```python
from build123d import *

# Parameters (mm, degrees)
SKETCH1_R            = 19
BOSS_EXTRUDE1_DEPTH  = 9.525
M5_CLEARANCE_HOLE1_D = 5.3


with BuildPart() as part:
    # Sketch1 → Boss-Extrude1 (new body)
    with BuildSketch(Plane.XY):
        with Locations(Location((0, 0, 0), (0, 0, 180))):
            Circle(SKETCH1_R)
    extrude(amount=BOSS_EXTRUDE1_DEPTH)

    # M5 Clearance Hole1 (through all)
    with Locations(Plane.XY.offset(9.525)):
        with Locations((-11.919791467, 6.881894812), (0, 13.763789624), (11.919791467, 6.881894812), (11.919791467, -6.881894812), (0, -13.763789624), (-11.919791467, -6.881894812)):
            Hole(M5_CLEARANCE_HOLE1_D / 2)


solid = part.part
```
Here's how the part is built. I have some questions about the finished solid (model axes, mm). Round coordinates to 2 decimals unless told otherwise and drop trailing zeros. Write each loop counter-clockwise with the first axis right and the second up, starting at its lowest first coordinate (ties: lowest second). Pieces come first, ordered by that corner, then holes.
Q1. Will these pins go through, and if not, where does the flat tip stop? P1, Ø5, axis at x = -11.92, y = 6.88, coming from the +Z side; P2, Ø1.5, axis at y = 4.5, z = 1, coming from the +X side; P3, Ø3, axis at y = 11.5, z = 3, coming from the -X side.
Q2. If we section it at B-B on z = 6: Write out the boundary of the cut face in (x, y).
Q3. If we mould it in two halves opening along Y, with no side actions, what happens to faces 1 (the cylindrical face through (4.119, 18.548, 4.696)), 2 (the flat face through (0, 0, 9.525)), 3 (the cylindrical face through (0.57, -16.35, 4.7))? For each: +Y half, -Y half, draft (parallel to the pull), parting line (faces both ways), or undercut.
Q4. If we section it at D-D on x = 8: Write out the boundary of the cut face in (y, z) (3 decimals), plus the area to 3 significant figures.
Q5. If we section it at C-C on x = -11: Write out the boundary of the cut face in (y, z) (3 decimals).
Q6. Please list where these lines run through material, in increasing order: probe 1 along Y at (x, z) = (0, 7); probe 2 along X at (y, z) = (9, 4.5); probe 3 along Y at (x, z) = (-10, 6.25).
Q7. If we section it at A-A on x = 0: Write out the boundary of the cut face in (y, z) (3 decimals), plus the area to 3 significant figures.
Answer below:
1. P1: passes through
1. P2: stops at x = 18.63
1. P3: stops at x = -16.16
2. outline: circle Ø38 at (0, 0); hole circle Ø5.3 at (-11.92, -6.88); hole circle Ø5.3 at (-11.92, 6.88); hole circle Ø5.3 at (0, -13.76); hole circle Ø5.3 at (0, 13.76); hole circle Ø5.3 at (11.92, -6.88); hole circle Ø5.3 at (11.92, 6.88)
3. face 1: parting line
3. face 2: draft
3. face 3: undercut
4. outline: (-17.234, 0) - (17.234, 0) - (17.234, 9.525) - (-17.234, 9.525) - close
4. area: 328 mm2
5. outline: (-15.492, 0) - (-9.367, 0) - (-9.367, 9.525) - (-15.492, 9.525) - close; (-4.397, 0) - (4.397, 0) - (4.397, 9.525) - (-4.397, 9.525) - close; (9.367, 0) - (15.492, 0) - (15.492, 9.525) - (9.367, 9.525) - close
6. probe 1: y = -19 to -16.41, -11.11 to 11.11, 16.41 to 19
6. probe 2: x = -16.73 to -13.51, -10.33 to 10.33, 13.51 to 16.73
6. probe 3: y = -16.16 to -8.71, -5.06 to 5.06, 8.71 to 16.16
7. outline: (-19, 0) - (-16.414, 0) - (-16.414, 9.525) - (-19, 9.525) - close; (-11.114, 0) - (11.114, 0) - (11.114, 9.525) - (-11.114, 9.525) - close; (16.414, 0) - (19, 0) - (19, 9.525) - (16.414, 9.525) - close
7. area: 261 mm2
